Build history of the part. All positions in model axes, mm. Give positions to 0.01 mm unless a question says otherwise; leave off trailing zeros. Write each loop counter-clockwise with the first axis right and the second up, starting at its lowest first coordinate (ties: lowest second). Pieces come first, ordered by that corner, then holes. Notation, with made-up numbers: (83.5, -39) - (107.5, -39) arc R37 cw to (107.5, -1) - close; hole circle Ø5 at (15.25, -10.75). An arc over 180 degrees is marked (long way). Use one line per item in the form item = value. Start each with the question number.
Autodesk Inventor part; units mm, degrees
ref_plane "YZ Plane" through (0, 0, 0) normal (1, 0, 0) x (0, 1, 0)
ref_plane "XZ Plane" through (0, 0, 0) normal (0, 1, 0) x (-1, 0, 0)
ref_plane "XY Plane" through (0, 0, 0) normal (0, 0, 1) x (1, 0, 0)
sketch "Sketch1" plane through (0, 0, 0) normal (0, 0, 1) x (1, 0, 0)
  line L0 (-34.9025, 5.6404) -> (104.7975, 5.6404)
  line L1 (104.7975, 5.6404) -> (104.7975, -26.3636)
  line L2 (104.7975, -26.3636) -> (-34.9025, -26.3636)
  line L3 (-34.9025, -26.3636) -> (-34.9025, 5.6404)
  point P0 (0, 0)
  dimension "d0" = 139.7
  dimension "d1" = 32.004
extrude "Extrusion1" add sketch "Sketch1" along normal blind 3.175
sketch "Sketch2" plane through (-34.9025, 5.6404, 0) normal (0, 1, 0) x (1, 0, 0)
  line L0 (0, -3.175) -> (139.7, -3.175)
  line L1 (139.7, 0) -> (139.7, -3.175)
  line L2 (0, 0) -> (139.7, 0)
  line L3 (0, 0) -> (0, -3.175)
  point P0 (34.9025, 0)
extrude "Extrusion2" add sketch "Sketch2" along normal blind 12.7
sketch "Sketch3" plane through (0, 0, 3.175) normal (0, 0, 1) x (1, 0, 0)
  line L0 (104.7975, -26.3636) -> (-34.9025, -26.3636)
  line L1 (-34.9025, 18.3404) -> (-15.8525, 18.3404)
  line L2 (-15.8525, 18.3404) -> (-15.8525, -26.3636)
  line L3 (-15.8525, -26.3636) -> (-34.9025, -26.3636)
  line L4 (-34.9025, -26.3636) -> (-34.9025, 18.3404)
  line L5 (-34.9025, -4.0116) -> (-25.3775, -4.0116)
  line L6 (-25.3775, -4.0116) -> (-25.3775, 2.3384)
  line L7 (-25.3775, 2.3384) -> (-34.9025, 2.3384)
  line L8 (-34.9025, 2.3384) -> (-34.9025, -4.0116)
  line L9 (-25.3775, -4.0116) -> (-25.3775, -10.3616)
  circle A0 centre (-25.3775, 2.3384) radius 1.9812
  circle A1 centre (-25.3775, -10.3616) radius 1.9812
  point P0 (0, 0)
  dimension "d6" = 19.05
  dimension "d7" = 6.35
  dimension "d8" = 6.35
  dimension "d9" = 3.9624
extrude "Extrusion3" cut sketch "Sketch3" against normal blind 12.7 contours A1 | A0 L6 L7 | L7 L6 A0
sketch "Sketch4" plane through (0, 0, 3.175) normal (0, 0, 1) x (1, 0, 0)
  line L0 (104.7975, 18.3404) -> (104.7975, -26.3636)
  line L1 (104.7975, -26.3636) -> (-34.9025, -26.3636)
  line L2 (104.7975, -4.0116) -> (96.7965, -4.0116)
  circle A0 centre (96.7965, -4.0116) radius 5.0038
  point P0 (0, 0)
  dimension "d12" = 8.001
  dimension "d13" = 10.0076
extrude "Extrusion4" cut sketch "Sketch4" against normal blind 12.7
sketch "Sketch5" plane through (0, 0, 3.175) normal (0, 0, 1) x (1, 0, 0)
  circle A0 centre (96.7965, -4.0116) radius 5.0038
  point P0 (0, 0)
extrude "Extrusion5" add sketch "Sketch5" against normal blind 3.175
sketch "Sketch6" plane through (0, 0, 3.175) normal (0, 0, 1) x (1, 0, 0)
  line L0 (104.7975, 18.3404) -> (104.7975, -26.3636)
  line L1 (104.7975, -26.3636) -> (-34.9025, -26.3636)
  line L2 (104.7975, -4.0116) -> (96.7975, -4.0116)
  circle A0 centre (96.7975, -4.0116) radius 5
  line L3 (103.3346, -4.0116) -> (73.3346, -4.0116)
  circle A1 centre (73.3346, -4.0116) radius 5
  point P0 (0, 0)
  dimension "d18" = 8
  dimension "d19" = 10
  dimension "d20" = 30
extrude "Extrusion6" cut sketch "Sketch6" against normal blind 3.175
sketch "Sketch7" plane through (0, 0, 3.175) normal (0, 0, 1) x (1, 0, 0)
  line L0 (-34.9025, -26.3636) -> (-34.9025, 18.3404)
  line L1 (104.7975, -26.3636) -> (-34.9025, -26.3636)
  line L2 (-34.9025, -4.0116) -> (-15.8525, -4.0116)
  line L3 (-15.8525, -4.0116) -> (52.9815, -4.0116)
  line L4 (52.9815, -4.0116) -> (44.8535, -4.0116)
  circle A0 centre (52.9815, -4.0116) radius 1.9812
  circle A1 centre (44.8535, -4.0116) radius 1.9812
  point P0 (0, 0)
  dimension "d23" = 19.05
  dimension "d24" = 68.834
  dimension "d25" = 8.128
  dimension "d26" = 3.9624
  dimension "d27" = 3.9624
extrude "Extrusion7" cut sketch "Sketch7" against normal blind 25.4
properties part number "linac connector bar"
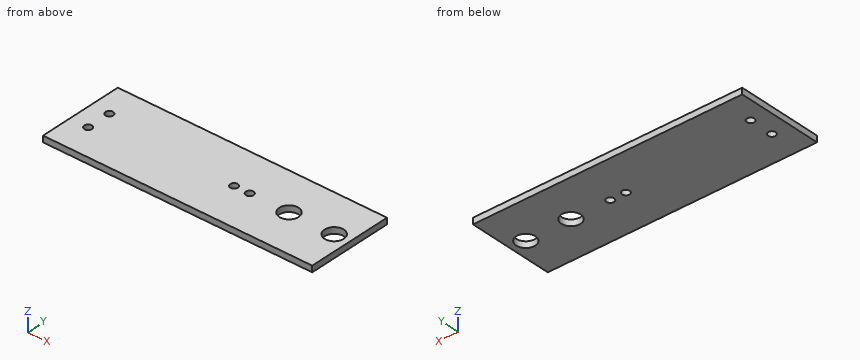
(1) Cut at A-A, the plane z = 1.3. Give the cut face in (x, y), then the cut area to 3 significant figures.
(2) Cut at C-C, the plane x = 45. Give the cut face in (y, z) (3 decimals).
(3) Pin check, flat tip, straight feed: pin 1 Ø3 at (x, y) = (-25.38, -10.36) entering from -Z. Stop position of the tip, or through.
(4) Cut at B-B, the plane x = 77. Give the cut face in (y, z) (3 decimals).
(5) Wall check: line 1 (X direction, y = -2.5, z = 0.2); line 2 (X direction, y = -2, z = 0.4) (1 decimal); line 3 (X direction, y = -10, z = 1.05). Give the ranges that are in metal, low to high. Write a range as from..to.
Solution:
q1.outline = (-34.9, -26.36) - (104.8, -26.36) - (104.8, 18.34) - (-34.9, 18.34) - close; hole circle Ø3.96 at (-25.38, -10.36); hole circle Ø3.96 at (-25.38, 2.34); hole circle Ø3.96 at (44.85, -4.01); hole circle Ø3.96 at (52.98, -4.01); hole circle Ø10 at (73.33, -4.01); hole circle Ø10 at (96.8, -4.01)
q1.area = 6,040 mm2
q2.outline = (-26.364, 0) - (-5.987, 0) - (-5.987, 3.175) - (-26.364, 3.175) - close; (-2.036, 0) - (18.34, 0) - (18.34, 3.175) - (-2.036, 3.175) - close
q3.pin_1 = through
q4.outline = (-26.364, 0) - (-7.412, 0) - (-7.412, 3.175) - (-26.364, 3.175) - close; (-0.611, 0) - (18.34, 0) - (18.34, 3.175) - (-0.611, 3.175) - close
q5.line_1 = -34.9..43.57, 46.13..51.7, 54.26..68.57, 78.1..92.03, 101.56..104.8
q5.line_2 = -34.9..68.8, 77.9..92.2, 101.4..104.8
q5.line_3 = -34.9..-27.33, -23.43..104.8
